Work out the finished part from the listing and answer in its coordinate system (mm). A direction names the side the tool comes from. Round coordinates to 2 decimals unless told otherwise and drop trailing zeros. Write each loop counter-clockwise with the first axis right and the second up, starting at its lowest first coordinate (ties: lowest second). Pieces come first, ordered by that corner, then holes.
from build123d import *

# Parameters (mm, degrees)
F1_DEPTH  = 63.5
F2_W      = 76.2
F2_H      = 4.7625
F3_DEPTH  = 103.378
F5_DEPTH  = 9.525
F6_W      = 57.15
F6_H      = 9.525
F7_DEPTH  = 6.35
F9_DEPTH  = 9.525
F10_W     = 76.2
F10_H     = 9.525
F11_DEPTH = 23.8125
F12_W     = 76.2
F12_H     = 9.525
F13_DEPTH = 46.0375
F15_DEPTH = 25.4
F17_DEPTH = 4.7625
F19_DEPTH = 54.356


with BuildPart() as f1:
    # F0 (on Front) → F1 (new body)
    with BuildSketch(Plane.XZ):
        Polygon((-48.8179810345, -18.3191206306), (-48.8179810345, -45.3066206306), (27.3820189655, -45.3066206306), (27.3820189655, -18.3191206306), (17.8570189655, -8.7941206306), (-39.2929810345, -8.7941206306), align=None)
    extrude(amount=F1_DEPTH)

    # F2 (on face) → F3 (cut)
    with BuildSketch(Plane.XZ.offset(63.5)):
        with Locations((-10.7179810345, -42.9253706306)):
            Rectangle(F2_W, F2_H)
    extrude(amount=-F3_DEPTH, mode=Mode.SUBTRACT)

    # F4 (on face) → F5 (join)
    with BuildSketch(Plane(origin=(0, 0, 0), x_dir=(-1, 0, 0), z_dir=(0, 1, 0))):
        Polygon((48.8179810345, -18.3191206306), (39.2929810345, -8.7941206306), (-17.8570189655, -8.7941206306), (-27.3820189655, -18.3191206306), (-27.3820189655, -40.5441206306), (48.8179810345, -40.5441206306), align=None)
    extrude(amount=F5_DEPTH)

    # F6 (on face) → F7 (join)
    with BuildSketch(Plane.XY.offset(-8.7941206306)):
        with Locations((-10.7179810345, 4.7625)):
            Rectangle(F6_W, F6_H)
    extrude(amount=F7_DEPTH)

    # F8 (on face) → F9 (join)
    with BuildSketch(Plane(origin=(0, 9.525, 0), x_dir=(-1, 0, 0), z_dir=(0, 1, 0))):
        Polygon((-17.8570189655, -8.7941206306), (-17.8570189655, -2.4441206306), (-27.3820189655, -2.4441206306), (-27.3820189655, -18.3191206306), align=None)
        Polygon((48.8179810345, -2.4441206306), (39.2929810345, -2.4441206306), (39.2929810345, -8.7941206306), (48.8179810345, -18.3191206306), align=None)
    extrude(amount=-F9_DEPTH)

    # F10 (on face) → F11 (join)
    with BuildSketch(Plane(origin=(0, 9.525, 0), x_dir=(-1, 0, 0), z_dir=(0, 1, 0))):
        with Locations((10.7179810345, -7.2066206306)):
            Rectangle(F10_W, F10_H)
    extrude(amount=F11_DEPTH)

    # F12 (on face) → F13 (join)
    with BuildSketch(Plane(origin=(0, 33.3375, 0), x_dir=(-1, 0, 0), z_dir=(0, 1, 0))):
        with Locations((10.7179810345, -7.2066206306)):
            Rectangle(F12_W, F12_H)
    extrude(amount=F13_DEPTH)

    # F14 (on face) → F15 (cut)
    with BuildSketch(Plane.XY.offset(-2.4441206306)):
        Polygon((-48.8179810345, 23.8125), (-15.4804810345, 79.375), (-48.8179810345, 79.375), align=None)
        Polygon((27.3820189655, 79.375), (-5.9554810345, 79.375), (27.3820189655, 23.8125), align=None)
    extrude(amount=-F15_DEPTH, mode=Mode.SUBTRACT)

    # F16 (on face) → F17 (join)
    with BuildSketch(Plane(origin=(0, 0, -40.5441206306), x_dir=(1, 0, 0), z_dir=(0, 0, -1))):
        Polygon((27.3820189655, 31.75), (27.3820189655, 42.0624), (-48.8179810345, 42.0624), (-48.8179810345, 21.43125), (27.3820189655, 21.43125), align=None)
    extrude(amount=F17_DEPTH)

    # F18 (on face) → F19 (cut)
    with BuildSketch(Plane.XY.offset(-8.7941206306)):
        with BuildLine():
            ThreePointArc((-10.7179810345, -46.0375), (-0.6151928983, -41.8527881362), (3.5695189655, -31.75))
            ThreePointArc((3.5695189655, -31.75), (-20.8207691707, -21.6472118638), (-10.7179810345, -46.0375))
        make_face()
    extrude(amount=-F19_DEPTH, mode=Mode.SUBTRACT)


solid = f1.part
Q1. A tool of negligible diameter and unlimited length cuts with its end or side. For faces 1 (the face through (-35, -21.431, -43)), 2 (the face through (22.553, -32.194, -13.49)), 3 (the face through (-35, -42.062, -43)), 4 (the face through (-44.1, -32.2, -13.6)), from which of +Z, -Z, +X, -X, +Y, -Y can it reach the whole face along a straight path? Write none if from no direction.
Q2. Find section D-D (y = 15). Determine the outline of the cut face in (x, z).
Q3. Find section A-A (y = -31.75). Determine the outline of the cut face in (x, z).
Q4. Given pin 1 (4 mm diameter, centred on x = 8, y = -35.5, fed in from +Z); pin 2 (2.5 mm diameter, centred on x = -38, z = -44, fed in from +Y); pin 3 (23.5 mm diameter, centred on x = -15.5, y = -56, fed in from -Z); pin 4 (6 mm diameter, centred on x = -34, y = 59, fed in from -Z), each flat-ended and moving along its own axis, determine where each tip first touches the part or whether it passes through.
Q5. Find the intervals of material crossed by L1, parallel to X at y = -32.5, z = -29; L2, parallel to X at y = -31.75, z = -26.5; L3, parallel to Y at x = -36, z = -16 (3 decimals), in increasing order.
Q6. The mould has two halves that part along Y. Classify faces 5 (the face through (-24.99, -31.12, -26.79)), 6 (the face through (-10, 0, -7)), 7 (the face through (-10, 30, -2.444)), 8 (the face through (13, -21.431, -43)): +Y half, -Y half, draft (parallel to the pull), parting line (faces both ways), or undercut.
Q7. Find section C-C (x = -17.5). Determine the outline of the cut face in (y, z) (3 decimals).
Report:
1. face 1: -Z, +X, -X, +Y
1. face 2: +Z, +X, -Y
1. face 3: -Z, +X, -X, -Y
1. face 4: +Z, -X, -Y
2. outline: (-48.82, -11.97) - (27.38, -11.97) - (27.38, -2.44) - (-48.82, -2.44) - close
3. outline: (-48.82, -45.31) - (-25.01, -45.31) - (-25.01, -8.79) - (-39.29, -8.79) - (-48.82, -18.32) - close; (3.57, -45.31) - (27.38, -45.31) - (27.38, -18.32) - (17.86, -8.79) - (3.57, -8.79) - close
4. pin 1: stops at z = -8.79
4. pin 2: stops at y = -21.43
4. pin 3: stops at z = -40.54
4. pin 4: passes through
5. L1: x = -48.82 to -24.99, 3.55 to 27.38
5. L2: x = -48.82 to -25.01, 3.57 to 27.38
5. L3: y = -63.5 to 9.525
6. face 5: undercut
6. face 6: -Y half
6. face 7: draft
6. face 8: +Y half
7. outline: (-63.5, -40.544) - (-44.325, -40.544) - (-44.325, -8.794) - (-63.5, -8.794) - close; (-19.175, -40.544) - (9.525, -40.544) - (9.525, -11.969) - (76.009, -11.969) - (76.009, -2.444) - (0, -2.444) - (0, -8.794) - (-19.175, -8.794) - close
